Build history of the part. All positions in model axes, mm. Face numbers are marked on the shaded views. A direction names the side the tool comes from. Give positions to 0.01 mm unless a question says otherwise; leave off trailing zeros. Write each loop counter-clockwise with the first axis right and the second up, starting at its lowest first coordinate (ties: lowest second). Pieces come first, ordered by that corner, then holes. Notation, with made-up numbers: (31.5, -0.5) -> (53.5, -0.5) arc R10 cw to (53.5, 16.5) -> close; hole circle Ø2 at (50.5, -12.75). An arc over 180 degrees is marked (long way). One line per question, with ' | ' between items. Start each with the question number.
(1) Band-saw the part on C-C, the plane y = -14.25. Give the cut face in (x, z), and give its area (3 significant figures).
(2) Pull direction X, two halves, no side cores. Call the marked faces 3, 4, 5 and 6: released by +X, released by -X, zero draft, split by the parting line, or undercut.
(3) Drill centre lines: probe 1 along Y at (x, z) = (19, 1.25); probe 2 along X at (y, z) = (-8.75, 14); probe 3 along X at (y, z) = (3.25, 14.75). Where is each one in solid material? Low to high. Write a range as from..to.
(4) Band-saw the part on D-D, the plane x = 13. Give the cut face in (y, z), and give its area (4 significant figures).
(5) Band-saw the part on A-A, the plane y = -3.5. Give the cut face in (x, z).
(6) Band-saw the part on B-B, the plane z = 15.5. Give the cut face in (x, y).
(7) Pin check, flat tips, straight feed: P1, Ø4, axis at y = -7, z = 10, coming from the -X side; P2, Ø6, axis at x = 15, y = -8.5, coming from the +Z side; P3, Ø1, axis at x = -3.5, z = 5.5, coming from the +Y side; P4, Ø4, axis at y = -6.5, z = 12.5, coming from the +X side. Stop position of each tip, or through.
(8) Tool access for the marked faces 1 and 2: list every direction of +Z, -Z, +X, -X, +Y, -Y with a clear straight run to the whole face (end or side of a thin tool).
from build123d import *

# Parameters (mm, degrees)
F0_W     = 60
F0_H     = 22.5
F1_DEPTH = 5
F2_W     = 35
F2_H     = 22.5
F3_DEPTH = 12.5
F5_DEPTH = 22.501
F6_R     = 2.5
F6_R_2   = 2.245551
F7_DEPTH = 5.001


with BuildPart() as f1:
    # F0 (on Top) → F1 (new body)
    with BuildSketch(Plane.XY):
        with Locations((-5.696384, -5.038032)):
            Rectangle(F0_W, F0_H)
    extrude(amount=F1_DEPTH)

    # F2 (on face) → F3 (join)
    with BuildSketch(Plane.XY.offset(5)):
        with Locations((-5.696384, -5.038032)):
            Rectangle(F2_W, F2_H)
    extrude(amount=F3_DEPTH)

    # F4 (on face) → F5 (cut, through all)
    with BuildSketch(Plane.XZ.offset(16.288032)):
        with BuildLine():
            Line((6.803616, 17.5), (-18.196384, 17.5))
            ThreePointArc((-18.196384, 17.5), (-5.696384, 5), (6.803616, 17.5))
        make_face()
    extrude(amount=-F5_DEPTH, mode=Mode.SUBTRACT)

    # F6 (on face) → F7 (cut, through all)
    with BuildSketch(Plane.XY.offset(5)):
        with Locations((-29.696384, -5.038232)):
            Circle(F6_R)
        with Locations((17.804456, -5.033552)):
            Circle(F6_R_2)
    extrude(amount=-F7_DEPTH, mode=Mode.SUBTRACT)


solid = f1.part
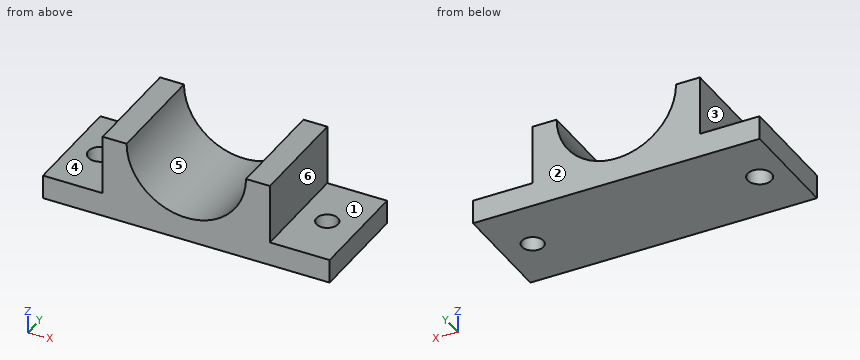
Results:
1) outline: (-35.7, 0) -> (24.3, 0) -> (24.3, 5) -> (11.8, 5) -> (11.8, 17.5) -> (6.8, 17.5) arc R12.5 cw to (-18.2, 17.5) -> (-23.2, 17.5) -> (-23.2, 5) -> (-35.7, 5) -> close | area: 492 mm²
2) face 3: released by -X | face 4: zero draft | face 5: undercut | face 6: released by +X
3) probe 1: y = -16.29..-6.93, -3.13..6.21 | probe 2: x = -23.2..-17.7, 6.3..11.8 | probe 3: x = -23.2..-17.89, 6.5..11.8
4) outline: (-16.29, 0) -> (6.21, 0) -> (6.21, 5) -> (-16.29, 5) -> close | area: 112.5 mm²
5) outline: (-35.7, 0) -> (-31.67, 0) -> (-31.67, 5) -> (-35.7, 5) -> close; (-27.73, 0) -> (16.16, 0) -> (16.16, 5) -> (11.8, 5) -> (11.8, 17.5) -> (6.8, 17.5) arc R12.5 cw to (-18.2, 17.5) -> (-23.2, 17.5) -> (-23.2, 5) -> (-27.73, 5) -> close; (19.44, 0) -> (24.3, 0) -> (24.3, 5) -> (19.44, 5) -> close
6) outline: (-23.2, -16.29) -> (-18.04, -16.29) -> (-18.04, 6.21) -> (-23.2, 6.21) -> close; (6.64, -16.29) -> (11.8, -16.29) -> (11.8, 6.21) -> (6.64, 6.21) -> close
7) P1: stops at x = -23.2 | P2: stops at z = 5 | P3: stops at y = 6.21 | P4: stops at x = 11.8
8) face 1: +Z, +X, +Y, -Y | face 2: +Z, -Z, +X, -X, +Y
